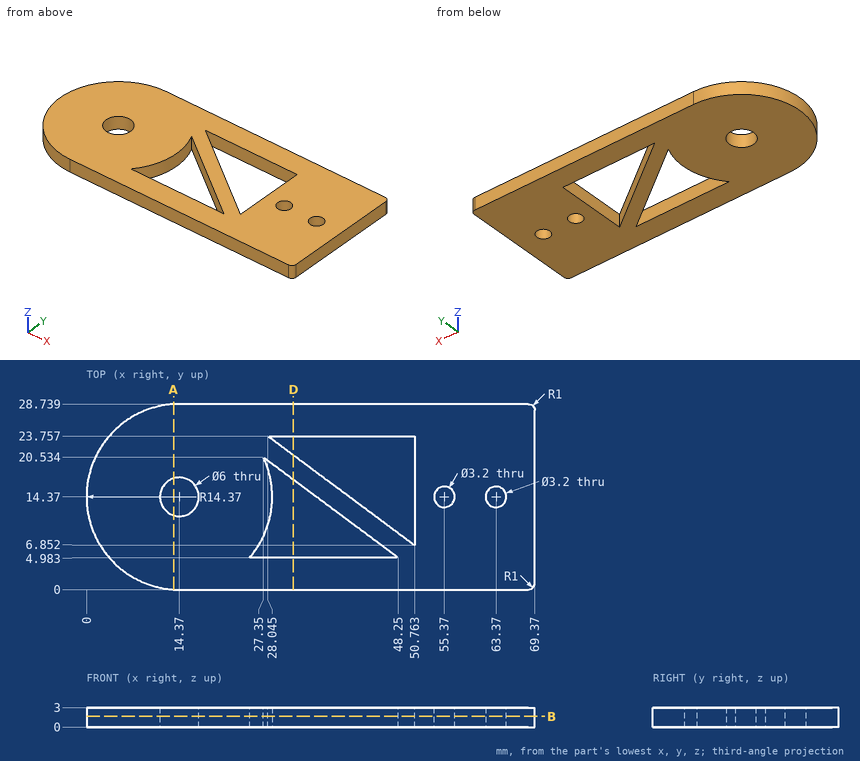
Study the drawing (mm; zero at the part's minimum x, y, z) and answer. Coordinates: 2 decimals unless noted, no trailing zeros. Loops run counter-clockwise (first coordinate to the right, second up) from the corner with the lowest first, then second, coordinate; pieces in that order, holes last. Notation, with made-up numbers: M 57,-33 L 101,-33 A22 ccw 101,-2 Z; hole C 36,81 d10. An arc over 180 degrees is marked long. Answer in a Markdown table with one row per item. Add a question column.
1. Find section B-B, the plane z = 1.65. State how many separate pieces and enclosed holes the cut face has, then the cut area to 3 significant figures.
2. Find section D-D, the plane x = 32. Write down the section's boundary in (y, z) (1 decimal).
3. Consider L1, parallel to Y at x = 63.5, z = 1.6 (1 decimal); L2, parallel to X at y = 14.25, z = 1.4 (1 decimal); L3, parallel to Y at x = 32, z = 2 (1 decimal). Determine where each line is inside the solid, lowest interval first.
4. Find section A-A, the plane x = 13.5. Write down the section's boundary in (y, z).
Reported:
| question | item | result |
|---|---|---|
| 1 | separate pieces | 1 |
| 1 | enclosed holes | 5 |
| 1 | area | 1,510 mm^2 |
| 2 | outline | M 0,0 L 5,0 L 5,3 L 0,3 Z; M 17.1,0 L 20.8,0 L 20.8,3 L 17.1,3 Z; M 23.8,0 L 28.7,0 L 28.7,3 L 23.8,3 Z |
| 3 | L1 | y = 0 to 12.8, 16 to 28.7 |
| 3 | L2 | x = 0 to 11.4, 17.4 to 28.7, 35.8 to 40.8, 50.8 to 53.8, 57 to 61.8, 65 to 69.4 |
| 3 | L3 | y = 0 to 5, 17.1 to 20.8, 23.8 to 28.7 |
| 4 | outline | M 0.03,0 L 11.5,0 L 11.5,3 L 0.03,3 Z; M 17.24,0 L 28.71,0 L 28.71,3 L 17.24,3 Z |
